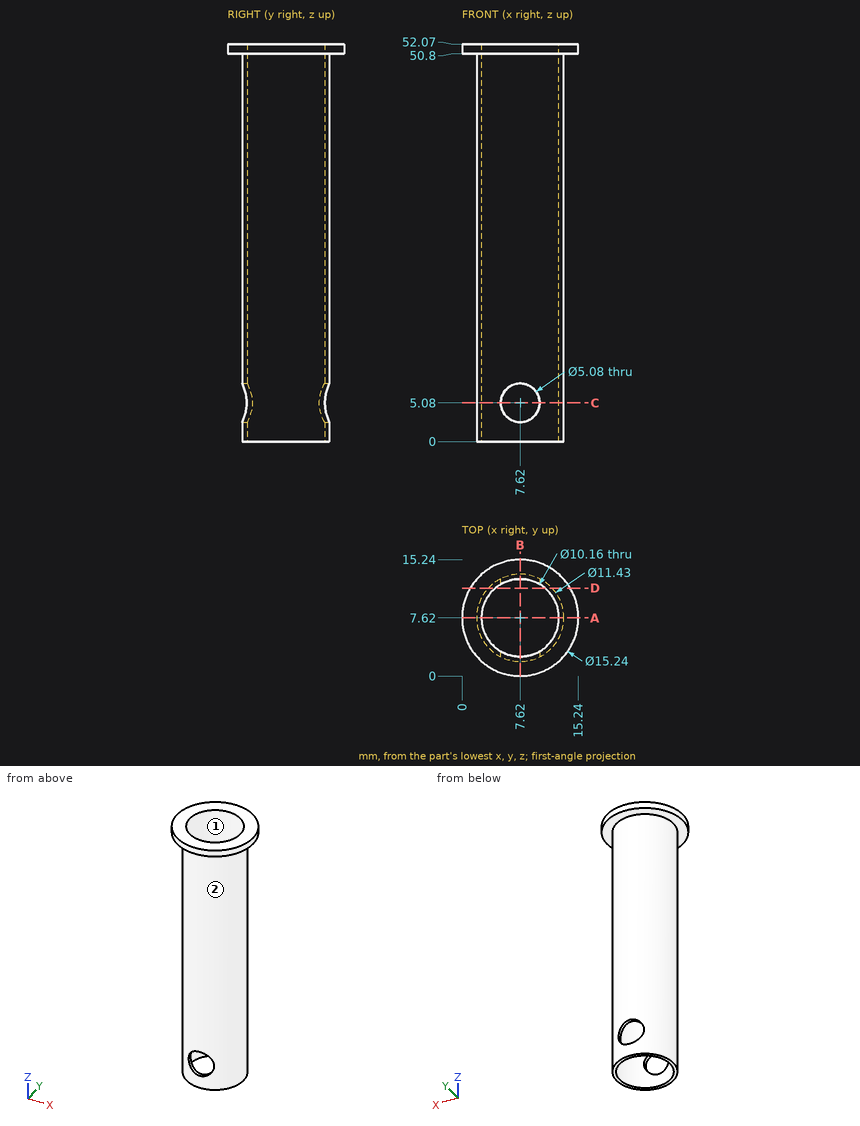
Part print with two shaded views. Sizes in mm from the minimum x, y, z corner. Coordinates: 2 decimals unless noted, no trailing zeros. Order: outer loops, then holes, each group sorted by start corner. A loop starts at its lowest first (then second) coordinate and runs counter-clockwise, first axis right, second up.
(1) Drill centre lines: L1, parallel to Y at x = 7.62, z = 22 (3 decimals); L2, parallel to Z at x = 7.62, y = 2.25; L3, parallel to Z at x = 1.25, y = 11.5. Where is each one in solid material? Low to high.
Solution:
L1: y = 1.905 to 2.54, 12.7 to 13.335
L2: z = 0 to 2.54, 7.62 to 52.07
L3: z = 50.8 to 52.07
(2) Saw through at B-B, the plane x = 7.62. Write the cut outline in (y, z) (3 decimals), and give its area (3 significant figures).
Solution:
outline: (0, 50.8) - (1.905, 50.8) - (1.905, 7.62) - (2.54, 7.62) - (2.54, 52.07) - (0, 52.07) - close; (1.905, 0) - (2.54, 0) - (2.54, 2.54) - (1.905, 2.54) - close; (12.7, 0) - (13.335, 0) - (13.335, 2.54) - (12.7, 2.54) - close; (12.7, 7.62) - (13.335, 7.62) - (13.335, 50.8) - (15.24, 50.8) - (15.24, 52.07) - (12.7, 52.07) - close
area: 64.5 mm2
(3) Saw through at A-A, the plane y = 7.62. Write the cut outline in (x, z) (3 decimals), and give its area (3 significant figures).
Solution:
outline: (0, 50.8) - (1.905, 50.8) - (1.905, 0) - (2.54, 0) - (2.54, 52.07) - (0, 52.07) - close; (12.7, 0) - (13.335, 0) - (13.335, 50.8) - (15.24, 50.8) - (15.24, 52.07) - (12.7, 52.07) - close
area: 71.0 mm2
(4) Pin check, flat tips, straight feed: pin 1 Ø4.5 at (x, y) = (10, 7.5) entering from -Z; pin 2 Ø1.5 at (x, y) = (12.5, 2.5) entering from -Z; pin 3 Ø6 at (x, z) = (7.62, 5.08) entering from +Y (3 decimals); pin 4 Ø6 at (x, z) = (2, 41.5) entering from -Y. Stop position of each tip, or through.
Solution:
pin 1: passes through
pin 2: stops at z = 50.8
pin 3: stops at y = 13.335
pin 4: stops at y = 2.54
(5) Saw through at D-D, the plane y = 11.5. Write the cut outline in (x, z), and give its area (3 significant figures).
Solution:
outline: (1.06, 50.8) - (3.42, 50.8) - (3.42, 0) - (4.34, 0) - (4.34, 52.07) - (1.06, 52.07) - close; (10.9, 0) - (11.82, 0) - (11.82, 50.8) - (14.18, 50.8) - (14.18, 52.07) - (10.9, 52.07) - close
area: 101 mm2
(6) Saw through at C-C, the plane z = 5.08. Write the cut outline in (x, y) (3 decimals).
Solution:
outline: (5.08, 2.5) - (5.08, 3.221) arc R5.08 cw to (5.08, 12.019) - (5.08, 12.74) arc R5.715 ccw to start; (10.16, 2.5) arc R5.715 ccw to (10.16, 12.74) - (10.16, 12.019) arc R5.08 cw to (10.16, 3.221) - close
(7) Mould opens along X. For the marked faces 1 and 2 say: released by +X, released by -X, zero draft, split by the parting line, or undercut.
Solution:
face 1: undercut
face 2: split by the parting line
